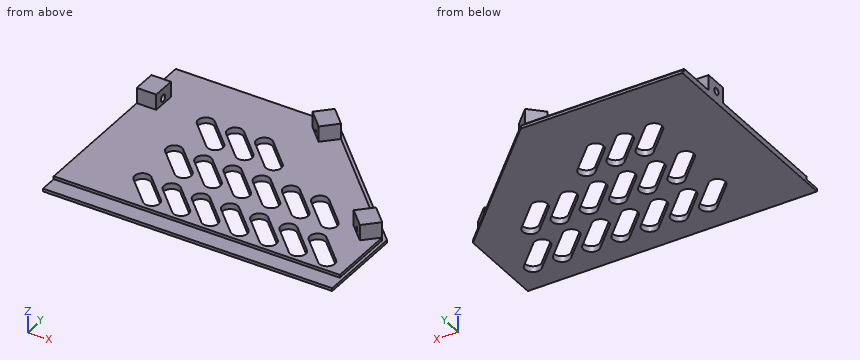
```python
from build123d import *

# Parameters (mm, degrees)
SALIENTE_EXTRUIR1_DEPTH = 1.5
SALIENTE_EXTRUIR2_DEPTH = 1.5
VENTILACION_DEPTH       = 3
MATRIZL1_COUNT          = 7
MATRIZL1_PITCH          = 15
MATRIZL1_COUNT_DIR2     = 3
MATRIZL1_PITCH_DIR2     = 26
CROQUIS4_W              = 10
CROQUIS4_H              = 12
SALIENTE_EXTRUIR3_DEPTH = 8
FIX_SUP_REACH           = 150.6
CROQUIS5_R              = 1.75
SALIENTE_EXTRUIR4_DEPTH = 8
CORTAR_EXTRUIR4_DEPTH   = 10
MATRIZL2_COUNT          = 2
MATRIZL2_PITCH          = 80


with BuildPart() as part:
    # Croquis1 → Saliente-Extruir1 (new body)
    with BuildSketch(Plane.XY):
        Polygon((74.3, 0), (-74.3, 0), (-74.3, 110.6), (8.7, 110.6), (74.3, 45), align=None)
    extrude(amount=SALIENTE_EXTRUIR1_DEPTH)

    # Croquis2 → Saliente-Extruir2 (add)
    with BuildSketch(Plane.XY.offset(1.5)):
        Polygon((-74.3, 109), (-74.3, 8.8), (72.7, 8.8), (72.7, 43.630151519), (7.330151519, 109), align=None)
    extrude(amount=SALIENTE_EXTRUIR2_DEPTH)

    # Croquis3 → ventilacion (cut)
    with BuildSketch(Plane.XY):
        with BuildLine():
            Line((52.128427125, 30.828427125), (65.128427125, 17.828427125))
            ThreePointArc((65.128427125, 17.828427125), (65.128427125, 12.171572875), (59.471572875, 12.171572875))
            Line((59.471572875, 12.171572875), (46.471572875, 25.171572875))
            ThreePointArc((46.471572875, 25.171572875), (46.471572875, 30.828427125), (52.128427125, 30.828427125))
        make_face()
    ventilacion = extrude(amount=VENTILACION_DEPTH, mode=Mode.SUBTRACT)

    # MatrizL1: ventilacion 7 × 3, 5 skipped
    with Locations(*[(-i * MATRIZL1_PITCH, j * MATRIZL1_PITCH_DIR2, 0) for i in range(MATRIZL1_COUNT) for j in range(MATRIZL1_COUNT_DIR2) if (i, j) not in ((0, 0), (0, 1), (0, 2), (1, 2), (2, 2), (3, 2))]):
        add(ventilacion, mode=Mode.SUBTRACT)

    # Croquis4 → Saliente-Extruir3 (add)
    with BuildSketch(Plane.XY.offset(3)):
        with Locations((-69.3, 83)):
            Rectangle(CROQUIS4_W, CROQUIS4_H)
    extrude(amount=SALIENTE_EXTRUIR3_DEPTH)

    # Croquis5 → fix-sup (cut, up to next)
    with BuildSketch(Plane.ZY.offset(74.3), mode=Mode.PRIVATE) as fix_sup_sk1:
        with Locations((6, 82.6)):
            Circle(CROQUIS5_R)
    fix_sup_tool1 = extrude(fix_sup_sk1.sketch, amount=-FIX_SUP_REACH, mode=Mode.PRIVATE) & part.part
    add(fix_sup_tool1.solids().sort_by_distance((-74.3, 82.6, 6))[0], mode=Mode.SUBTRACT)

    # Croquis6 → Saliente-Extruir4 (add)
    with BuildSketch(Plane.XY.offset(3)):
        Polygon((72.7, 43.630151519), (64.214718626, 52.115432893), (57.143650814, 45.044365081), (65.628932188, 36.559083707), align=None)
    saliente_extruir4 = extrude(amount=SALIENTE_EXTRUIR4_DEPTH)

    # Croquis7 → Cortar-Extruir4 (cut)
    with BuildSketch(Plane(origin=(58.16507576, 58.16507576, 0), x_dir=(0, 0, -1), z_dir=(0.707106781, 0.707106781, 0))):
        Polygon((-4.35, -13.429653964), (-6.3, -14.555486989), (-4.35, -15.681320014), align=None)
    cortar_extruir4 = extrude(amount=-CORTAR_EXTRUIR4_DEPTH, mode=Mode.SUBTRACT)

    # MatrizL2: Saliente-Extruir4, Cortar-Extruir4 ×2
    with Locations(*[Vector(-0.707106781, 0.707106781, 0) * (i * MATRIZL2_PITCH) for i in range(1, MATRIZL2_COUNT)]):
        add(saliente_extruir4)
        add(cortar_extruir4, mode=Mode.SUBTRACT)


solid = part.part
```
Verification items for the finished model (mm, model axes). Round coordinates to 2 decimals unless told otherwise and drop trailing zeros. Answer as a JSON object with one key per item and string values. Group by question number.
Q1. Go/stop test with flat-tipped pins: pin 1 Ø6.5 at (x, z) = (-68, 9) entering from -Y; pin 2 Ø4 at (x, y) = (37, 58) entering from +Z; pin 3 Ø1.2 at (x, z) = (-47, 2.5) entering from +Y. Record where each tip stops, or that it passes through.
Q2. Section check A-A, the plane y = 15. Give the number of separate pieces and of enclosed holes in the cut face, plus the area to 3 significant figures.
Q3. Thickness scan on line 1 (Z direction, x = -66, y = 82); line 2 (Z direction, x = -70.5, y = 82.6); line 3 (Y direction, x = 45, z = 2.5). Record the ranges inside material, lowest first.
Found:
{
 "1": {"pin 1": "stops at y = 77", "pin 2": "stops at z = 3", "pin 3": "stops at y = 109"},
 "2": {"separate pieces": "8", "enclosed holes": "0", "area": "241 mm^2"},
 "3": {"line 1": "z = 0 to 4.36, 7.64 to 11", "line 2": "z = 0 to 4.25, 7.75 to 11", "line 3": "y = 8.8 to 11.73, 22.96 to 37.73, 48.96 to 71.33"}
}
